Verification items for the finished model (mm, model axes). Coordinates: 2 decimals unless noted, no trailing zeros. Loops run counter-clockwise (first coordinate to the right, second up) from the corner with the lowest first, then second, coordinate; pieces in that order, holes last. Notation, with made-up numbers: (74.25, 27) -> (118.25, 27) arc R30 ccw to (118.25, 55) -> close; hole circle Ø11 at (10.5, 62). An arc over 180 degrees is marked (long way). Use CSV: the item, a comma, the result in double quotes. Start each with the question number.
```python
from build123d import *

# Parameters (mm, degrees)
CROQUIS1_R            = 45
DISCO_DEPTH           = 5
PATR_NGIRO_DEPTH      = 64.835726674
CROQUIS7_R            = 1.5875
BARRENOSEJES_DEPTH    = 10
CROQUIS8_R            = 3.5
CORTAR_EXTRUIR5_DEPTH = 2.5


with BuildPart() as part:
    # Croquis1 → Disco (new body)
    with BuildSketch(Plane.XY):
        Circle(CROQUIS1_R)
    extrude(amount=DISCO_DEPTH)

    # Croquis6 → PatrónGiro (cut, through all)
    with BuildSketch(Plane.XY.offset(5)):
        with BuildLine():
            ThreePointArc((-30.527395483, -17.625), (-4.464035413, -25.86746934), (6.062177826, -0.639788633))
            ThreePointArc((6.062177826, -0.639788633), (18.906715666, 0.249805468), (21.434128744, -12.375))
            ThreePointArc((21.434128744, -12.375), (23.355762114, -19.54663337), (30.527395483, -17.625))
            ThreePointArc((30.527395483, -17.625), (24.633903286, 9.067766599), (-2.477015704, 5.569894316))
            ThreePointArc((-2.477015704, 5.569894316), (-9.669695714, 16.248793335), (0, 24.75))
            ThreePointArc((0, 24.75), (5.25, 30), (0, 35.25))
            ThreePointArc((0, 35.25), (-20.169867874, 16.799702741), (-3.585162122, -4.930105684))
            ThreePointArc((-3.585162122, -4.930105684), (-9.237019952, -16.498598803), (-21.434128744, -12.375))
            ThreePointArc((-21.434128744, -12.375), (-28.605762114, -10.45336663), (-30.527395483, -17.625))
        make_face()
    extrude(amount=-PATR_NGIRO_DEPTH, mode=Mode.SUBTRACT)

    # Croquis7 → BarrenosEjes (cut)
    with BuildSketch(Plane.XY.offset(5)):
        with Locations((-29.5, 0)):
            Circle(CROQUIS7_R)
        with Locations((14.75, 25.547749412)):
            Circle(CROQUIS7_R)
        with Locations((14.75, -25.547749412)):
            Circle(CROQUIS7_R)
    extrude(amount=-BARRENOSEJES_DEPTH, mode=Mode.SUBTRACT)

    # Croquis8 → Cortar-Extruir5 (cut)
    with BuildSketch(Plane.XY.offset(5)):
        with Locations((-29.5, 0)):
            Circle(CROQUIS8_R)
        with Locations((14.75, -25.547749412)):
            Circle(CROQUIS8_R)
        with Locations((14.75, 25.547749412)):
            Circle(CROQUIS8_R)
    extrude(amount=-CORTAR_EXTRUIR5_DEPTH, mode=Mode.SUBTRACT)


solid = part.part
```
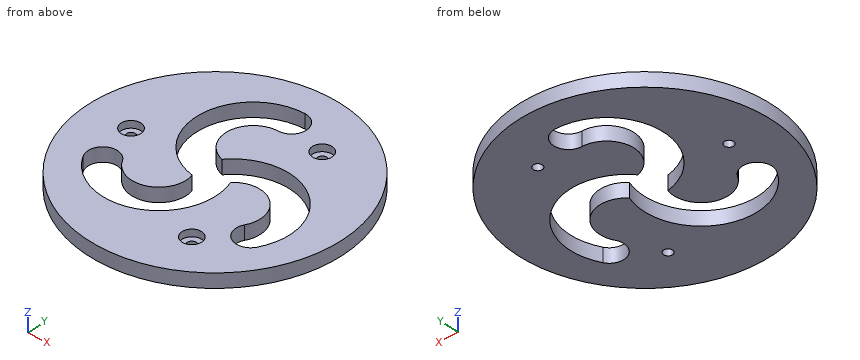
1. Depth check by flat-ended pin: pin 1 (3 mm diameter, centred on y = 18.5, z = 4.5, fed in from +X); pin 2 (5 mm diameter, centred on x = 14.75, y = 25.55, fed in from -Z); pin 3 (2 mm diameter, centred on x = -23, z = 3.5, fed in from +Y); pin 4 (5 mm diameter, centred on x = -29.5, y = 0, fed in from +Z). Enter the tip coordinate at first touch or a pass-through.
2. Cross-section at B-B, the plane y = -15. Record the boundary of the cut face in (x, z), plus the area to 3 significant figures.
3. Scan lines: line 1 (X direction, y = -24, z = 3.65); line 2 (X direction, y = -13.5, z = 1.5); line 3 (X direction, y = -7, z = 0.3). Record each from-to range of solid material in increasing order.
4. Cross-section at A-A, the plane x = 14.75. Record the boundary of the cut face in (y, z).
5. Cross-section at C-C, the plane x = -7.5. Record the boundary of the cut face in (y, z), plus the area to 3 significant figures.
6. Cross-section at D-D, the plane y = 38. Record the boundary of the cut face in (x, z).
Solution:
1,pin 1,"stops at x = 41.67"
1,pin 2,"stops at z = 0"
1,pin 3,"stops at y = 39.26"
1,pin 4,"stops at z = 2.5"
2,outline,"(-42.43, 0) -> (-31.23, 0) -> (-31.23, 5) -> (-42.43, 5) -> close; (-19.22, 0) -> (-6.76, 0) -> (-6.76, 5) -> (-19.22, 5) -> close; (5.82, 0) -> (20.73, 0) -> (20.73, 5) -> (5.82, 5) -> close; (31.8, 0) -> (42.43, 0) -> (42.43, 5) -> (31.8, 5) -> close"
2,area,"246 mm2"
3,line 1,"x = -38.07 to -24.73, -1.25 to 11.61, 17.89 to 38.07"
3,line 2,"x = -42.93 to -31.01, -20.68 to -5.31, 6.35 to 20.95, 32.33 to 42.93"
3,line 3,"x = -44.45 to -3.25, 7.25 to 22.73, 33.23 to 44.45"
4,outline,"(-42.51, 0) -> (-27.14, 0) -> (-27.14, 2.5) -> (-29.05, 2.5) -> (-29.05, 5) -> (-42.51, 5) -> close; (-23.96, 0) -> (2.09, 0) -> (2.09, 5) -> (-22.05, 5) -> (-22.05, 2.5) -> (-23.96, 2.5) -> close; (12.67, 0) -> (23.96, 0) -> (23.96, 2.5) -> (22.05, 2.5) -> (22.05, 5) -> (12.67, 5) -> close; (27.14, 0) -> (42.51, 0) -> (42.51, 5) -> (29.05, 5) -> (29.05, 2.5) -> (27.14, 2.5) -> close"
5,outline,"(-44.37, 0) -> (-26.99, 0) -> (-26.99, 5) -> (-44.37, 5) -> close; (-15.56, 0) -> (-3.81, 0) -> (-3.81, 5) -> (-15.56, 5) -> close; (8.77, 0) -> (21.23, 0) -> (21.23, 5) -> (8.77, 5) -> close; (33.81, 0) -> (44.37, 0) -> (44.37, 5) -> (33.81, 5) -> close"
5,area,"261 mm2"
6,outline,"(-24.1, 0) -> (24.1, 0) -> (24.1, 5) -> (-24.1, 5) -> close"
